Could you check a few things on this drawing? It's one solid part, dimensions in mm from its lowest x, y, z. Round coordinates to 2 decimals unless told otherwise and drop trailing zeros. Order: outer loops, then holes, each group sorted by start corner. A loop starts at its lowest first (then second) coordinate and runs counter-clockwise, first axis right, second up. Notation, with made-up numbers: (-34.75, -39.75) -> (-30.75, -39.75) arc R30 ccw to (-30.75, -3.75) -> close; hole circle Ø2 at (35, 62). An arc over 180 degrees is marked (long way). Use a Markdown table: item, result. Add a question column.
(1) I want a section at C-C, the plane z = 1.1. Please give me the cut outline in (x, y), then the cut area to 3 significant figures.
(2) If I drill on probe 1 along Y at (x, z) = (6, 1.3); probe 2 along X at (y, z) = (51, 0.7); probe 3 along X at (y, z) = (52, 0.75), over which ranges is the centre line in solid material (lowest first)?
(3) I want a section at B-B, the plane x = 6. Please give me the cut outline in (y, z).
(4) I want a section at A-A, the plane y = 54. Please give me the cut outline in (x, z), then the cut area to 3 significant figures.
(5) I want a section at D-D, the plane y = 21. Please give me the cut outline in (x, z).
(6) I'm going to push flat-ended pins straight in: P1, Ø0.9, axis at y = 8, z = 1.5, coming from the +X side; P2, Ø1.5, axis at x = 64, z = 1.5, coming from the -Y side. Where does each tip first touch, or does it pass through?
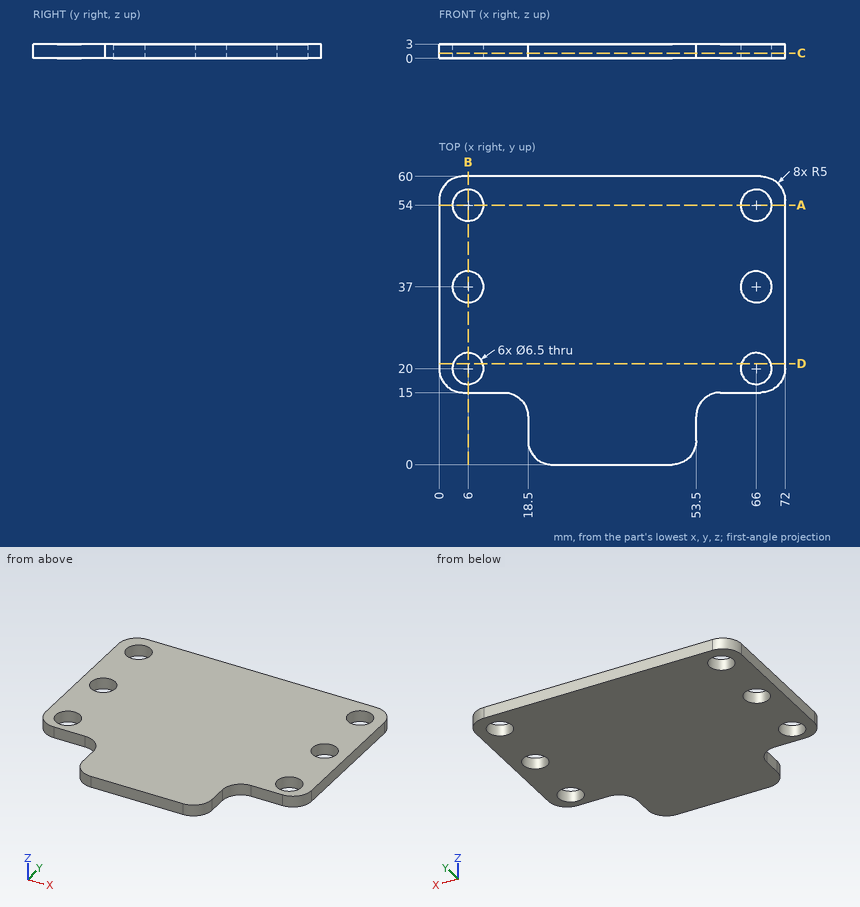
Taken from the geometry:
| question | item | result |
|---|---|---|
| 1 | outline | (0, 20) arc R5 ccw to (5, 15) -> (13.5, 15) arc R5 cw to (18.5, 10) -> (18.5, 5) arc R5 ccw to (23.5, 0) -> (48.5, 0) arc R5 ccw to (53.5, 5) -> (53.5, 10) arc R5 cw to (58.5, 15) -> (67, 15) arc R5 ccw to (72, 20) -> (72, 55) arc R5 ccw to (67, 60) -> (5, 60) arc R5 ccw to (0, 55) -> close; hole circle Ø6.5 at (6, 20); hole circle Ø6.5 at (6, 37); hole circle Ø6.5 at (6, 54); hole circle Ø6.5 at (66, 20); hole circle Ø6.5 at (66, 37); hole circle Ø6.5 at (66, 54) |
| 1 | area | 3,540 mm2 |
| 2 | probe 1 | y = 15 to 16.75, 23.25 to 33.75, 40.25 to 50.75, 57.25 to 60 |
| 2 | probe 2 | x = 0 to 4.75, 7.25 to 64.75, 67.25 to 72 |
| 2 | probe 3 | x = 0 to 3.44, 8.56 to 63.44, 68.56 to 72 |
| 3 | outline | (15, 0) -> (16.75, 0) -> (16.75, 3) -> (15, 3) -> close; (23.25, 0) -> (33.75, 0) -> (33.75, 3) -> (23.25, 3) -> close; (40.25, 0) -> (50.75, 0) -> (50.75, 3) -> (40.25, 3) -> close; (57.25, 0) -> (60, 0) -> (60, 3) -> (57.25, 3) -> close |
| 4 | outline | (0, 0) -> (2.75, 0) -> (2.75, 3) -> (0, 3) -> close; (9.25, 0) -> (62.75, 0) -> (62.75, 3) -> (9.25, 3) -> close; (69.25, 0) -> (72, 0) -> (72, 3) -> (69.25, 3) -> close |
| 4 | area | 177 mm2 |
| 5 | outline | (0, 0) -> (2.91, 0) -> (2.91, 3) -> (0, 3) -> close; (9.09, 0) -> (62.91, 0) -> (62.91, 3) -> (9.09, 3) -> close; (69.09, 0) -> (72, 0) -> (72, 3) -> (69.09, 3) -> close |
| 6 | P1 | stops at x = 53.5 |
| 6 | P2 | stops at y = 15 |
